Work out the finished part from the listing and answer in its coordinate system (mm). A direction names the side the tool comes from. Coordinates: 2 decimals unless noted, no trailing zeros. Write each loop counter-clockwise with the first axis right and the second up, starting at its lowest first coordinate (ties: lowest second). Pieces come first, ordered by that corner, then holes. Notation, with made-up numbers: M 63.5,2 L 90.5,2 A23 ccw 90.5,22 Z; hole C 67,-36.5 d2. An arc over 180 degrees is marked long. Use CSV: the item, a comma, the result in double quotes.
from build123d import *

# Parameters (mm, degrees)
BOSS_EXTRUDE1_START   = -224
BOSS_EXTRUDE1_DEPTH   = 224
BOSS_EXTRUDE2_DEPTH   = 6.35
BOSS_EXTRUDE3_DEPTH   = 5
M12_CLEARANCE_HOLE1_D = 13.5
FILLET1_R             = 10
MIRROR1_COPY_1_DEPTH  = 5
FILLET1_OF_MIRROR1_R  = 10


with BuildPart() as part:
    # Sketch12 → Revolve1 (revolve)
    with BuildSketch(Plane.XY, mode=Mode.PRIVATE) as revolve1_sk:
        Polygon((-25.4, 0), (-25.4, 254), (-21.22866, 254), (-21.22866, 127), (-21.22866, 0), align=None)
    revolve(revolve1_sk.sketch.rotate(Axis((0, 0, 0), (0, 1, 0)), 270), axis=Axis((0, 0, 0), (0, 1, 0)))

    # Sketch14 → Boss-Extrude1 (add)
    with BuildSketch(Plane(origin=(0, 30, 0), x_dir=(-1, 0, 0), z_dir=(0, -1, 0)).offset(BOSS_EXTRUDE1_START)):
        with BuildLine():
            Line((-25.4, 0), (-25.4, -25.4))
            Line((-25.4, -25.4), (-3.2e-08, -25.4))
            ThreePointArc((-3.2e-08, -25.4), (-17.960512254, -17.960512231), (-25.4, 0))
        make_face()
        with BuildLine():
            ThreePointArc((25.4, 0), (17.960512231, -17.960512254), (-3.2e-08, -25.4))
            Line((-3.2e-08, -25.4), (25.4, -25.4))
            Line((25.4, -25.4), (25.4, 0))
        make_face()
    extrude(amount=BOSS_EXTRUDE1_DEPTH)

    # Sketch27 → Boss-Extrude2 (add)
    with BuildSketch(Plane.XY.offset(25.4)):
        Polygon((25.4, 254), (25.4, 30), (53.4, 30), (53.4, 75), (35.4, 106.176914536), (35.4, 177.823085464), (53.4, 209), (53.4, 254), align=None)
    boss_extrude2 = extrude(amount=-BOSS_EXTRUDE2_DEPTH)

    # Sketch32 → Boss-Extrude3 (add)
    with BuildSketch(Plane(origin=(0, 65, 0), x_dir=(-1, 0, 0), z_dir=(0, -1, 0))):
        Polygon((-53.4, -19.05), (-25.4, -19.05), (-25.4, 0), align=None)
    boss_extrude3 = extrude(amount=-BOSS_EXTRUDE3_DEPTH)

    # Mirror2: Boss-Extrude3 across plane
    add(boss_extrude3.mirror(Plane(origin=(0, 142, 0), x_dir=(0, 0, 1), z_dir=(0, -1, 0))))

    # M12 Clearance Hole1 (through all)
    with Locations(Plane.XY.offset(25.4)):
        with Locations((39.4, 46), (39.4, 238)):
            m12_clearance_hole1 = Hole(M12_CLEARANCE_HOLE1_D / 2)

    # Fillet1
    fillet1_edges = [part.edges().sort_by_distance(p)[0] for p in [
        (53.4, 254, 22.225),
        (53.4, 209, 22.225),
        (35.4, 177.823085464, 22.225),
        (35.4, 106.176914536, 22.225),
        (53.4, 75, 22.225),
        (53.4, 30, 22.225),
    ]]
    fillet(fillet1_edges, radius=FILLET1_R)

    # Mirror1: Boss-Extrude2, Boss-Extrude3, M12 Clearance Hole1 across plane
    add(boss_extrude2.mirror(Plane(origin=(0, 0, 0), x_dir=(0, 0, 1), z_dir=(1, 0, 0))))
    add(boss_extrude3.mirror(Plane(origin=(0, 0, 0), x_dir=(0, 0, 1), z_dir=(1, 0, 0))))
    add(m12_clearance_hole1.mirror(Plane(origin=(0, 0, 0), x_dir=(0, 0, 1), z_dir=(1, 0, 0))), mode=Mode.SUBTRACT)

    # Mirror1 copy 1 sketch → Mirror1 copy 1 (add)
    with BuildSketch(Plane(origin=(0, 219, 0), x_dir=(1, 0, 0), z_dir=(0, 1, 0))):
        Polygon((-53.4, -19.05), (-25.4, -19.05), (-25.4, 0), align=None)
    extrude(amount=-MIRROR1_COPY_1_DEPTH)

    # Fillet1 of Mirror1
    fillet1_of_mirror1_edges = [part.edges().sort_by_distance(p)[0] for p in [
        (-53.4, 254, 22.225),
        (-53.4, 209, 22.225),
        (-35.4, 177.823085464, 22.225),
        (-35.4, 106.176914536, 22.225),
        (-53.4, 75, 22.225),
        (-53.4, 30, 22.225),
    ]]
    fillet(fillet1_of_mirror1_edges, radius=FILLET1_OF_MIRROR1_R)


solid = part.part
Item 1: The part is cut by section D-D (y = 201). Write down the section's boundary in (x, z), then the cut area to 3 significant figures.
Answer:
outline,"M -48.78,19.05 L -25.4,19.05 L -25.4,0 A25.4 ccw 25.4,0 L 25.4,19.05 L 48.78,19.05 L 48.78,25.4 L -48.78,25.4 Z; hole C 0,0 d42.46"
area,"1,180 mm2"
Item 2: For a pull along Y with two mould halves and no side action, classify faces 1 (the face through (50.39, 251.15, 22.18)), 2 (the face through (-25.4, 48, 10)), 3 (the face through (33, 70, 14)) as released by +Y, released by -Y, zero draft, split by the parting line, or undercut.
Answer:
face 1,"released by +Y"
face 2,"zero draft"
face 3,"undercut"
Item 3: The part is cut by section A-A (y = 238). Write down the section's boundary in (x, z), then the cut area to 3 significant figures.
Answer:
outline,"M -53.4,19.05 L -46.15,19.05 L -46.15,25.4 L -53.4,25.4 Z; M -32.65,19.05 L -25.4,19.05 L -25.4,0 A25.4 ccw 25.4,0 L 25.4,19.05 L 32.65,19.05 L 32.65,25.4 L -32.65,25.4 Z; M 46.15,19.05 L 53.4,19.05 L 53.4,25.4 L 46.15,25.4 Z; hole C 0,0 d42.46"
area,"1,070 mm2"
Item 4: A tool of negligible diameter and unlimited length cuts with its end or side. For faces 4 (the face through (-33, 233, 19.05)), 5 (the face through (-33, 214, 14)), 6 (the face through (-26, 30, 20)), 7 (the face through (-53.07, 74.87, 22.18)), from which of +Z, -Z, +X, -X, +Y, -Y can it reach the whole face along a straight path? Write none if from no direction.
Answer:
face 4,"-Z, -X, +Y"
face 5,"-Z, -X"
face 6,"+Z, -X, -Y"
face 7,"+Z, -Z, -X"
Item 5: Given pin 1 (15 mm diameter, centred on y = 111, z = 5.5, fed in from -X); pin 2 (15 mm diameter, centred on x = 44.5, z = 11.5, fed in from +Y); pin 3 (21 mm diameter, centred on x = 42.5, z = 14, fed in from -Y), each flat-ended and moving along its own axis, determine where each tip first touches the part or whether it passes through.
Answer:
pin 1,"stops at x = -25.4"
pin 2,"stops at y = 219"
pin 3,"stops at y = 30"
Item 6: The part is cut by section B-B (x = 39.4). Write down the section's boundary in (y, z) (3 decimals).
Answer:
outline,"M 30,19.05 L 39.25,19.05 L 39.25,25.4 L 30,25.4 Z; M 52.75,19.05 L 65,19.05 L 65,9.525 L 70,9.525 L 70,19.05 L 99.249,19.05 L 99.249,25.4 L 52.75,25.4 Z; M 184.751,19.05 L 214,19.05 L 214,9.525 L 219,9.525 L 219,19.05 L 231.25,19.05 L 231.25,25.4 L 184.751,25.4 Z; M 244.75,19.05 L 254,19.05 L 254,25.4 L 244.75,25.4 Z"
Item 7: Consider probe 1 along X at (y, z) = (204, 0.5); probe 2 along Y at (x, z) = (38, 19); probe 3 along Y at (x, z) = (39, 23). Determine where each line is inside the solid, lowest interval first.
Answer:
probe 1,"x = -25.4 to -21.22, 21.22 to 25.4"
probe 2,"y = 65 to 70, 214 to 219"
probe 3,"y = 30 to 39.26, 52.74 to 99.94, 184.06 to 231.26, 244.74 to 254"
Item 8: The part is cut by section C-C (z = 16). Write down the section's boundary in (x, y), then the cut area to 3 significant figures.
Answer:
outline,"M -48.92,65 L -25.4,65 L -25.4,30 L -19.73,30 L -19.73,0 L -13.95,0 L -13.95,254 L -25.4,254 L -25.4,219 L -48.92,219 L -48.92,214 L -25.4,214 L -25.4,70 L -48.92,70 Z; M 13.95,0 L 19.73,0 L 19.73,30 L 25.4,30 L 25.4,65 L 48.92,65 L 48.92,70 L 25.4,70 L 25.4,214 L 48.92,214 L 48.92,219 L 25.4,219 L 25.4,254 L 13.95,254 Z"
area,"5,950 mm2"
